```python
from build123d import *

# Parameters (mm, degrees)
THICKEN1_T2                     = 2
SURFACE_EXTRUDE1_2_DEPTH        = 65
THICKEN2_T1                     = 2
BOSS_EXTRUDE2_REACH             = 83.701
BOSS_EXTRUDE2_END_MAJOR_RADIUS  = 15
BOSS_EXTRUDE2_END_MINOR_RADIUS  = 18
BOSS_EXTRUDE2_DIRECTION_2_DEPTH = 65
SKETCH5_R                       = 1
CUT_EXTRUDE2_DEPTH              = 65
SURFACE_EXTRUDE2_3_DEPTH        = 5
THICKEN3_T1                     = 1


with BuildPart() as body_1:
    # Surface-Revolve1: a surface, the sketch's curves turned about an axis
    with BuildLine(Plane(origin=(0, 0, 0), x_dir=(1, 0, 0), z_dir=(0, 1, 0)), mode=Mode.PRIVATE) as surface_revolve1_1_path:
        Line((0, 0), (0, 15))
        ThreePointArc((0, 15), (5.857864376, 29.142135624), (20, 35))
    surface_revolve1_1 = Shell.revolve(surface_revolve1_1_path.wire(), 360, Axis((0, 0, 0), (1, 0, 0)))
    add(Solid.thicken(surface_revolve1_1, -THICKEN1_T2))

    # Surface-Extrude1: a surface, the sketch's curves swept straight by 65 mm
    with BuildLine(Plane(origin=(20, 0, 0), x_dir=(0, 0, -1), z_dir=(1, 0, 0)), mode=Mode.PRIVATE) as surface_extrude1_2_path:
        CenterArc((0, 0), 35, 0, 360)
    surface_extrude1_2 = Shell.extrude(surface_extrude1_2_path.wire(), (1 * SURFACE_EXTRUDE1_2_DEPTH, 0 * SURFACE_EXTRUDE1_2_DEPTH, 0 * SURFACE_EXTRUDE1_2_DEPTH))
    add(Solid.thicken(surface_extrude1_2, THICKEN2_T1))

    # Boss-Extrude2: up to this torus (the profile starts inside it)
    boss_extrude2_end = Plane(origin=(20, 0, 0), z_dir=(1, 0, 0)) * Torus(BOSS_EXTRUDE2_END_MAJOR_RADIUS, BOSS_EXTRUDE2_END_MINOR_RADIUS, mode=Mode.PRIVATE)
    # Sketch2 → Boss-Extrude2 (add, up to the surface)
    with BuildSketch(Plane(origin=(20, 0, 0), x_dir=(0, 0, -1), z_dir=(1, 0, 0)), mode=Mode.PRIVATE) as boss_extrude2_sk1:
        with BuildLine():
            Line((-2, 31), (-2, 33))
            Line((-2, 33), (2, 33))
            Line((2, 33), (2, 31))
            ThreePointArc((2, 31), (0, 29), (-2, 31))
        make_face()
    boss_extrude2_tool1 = extrude(boss_extrude2_sk1.sketch, amount=-BOSS_EXTRUDE2_REACH, mode=Mode.PRIVATE) & boss_extrude2_end
    add(boss_extrude2_tool1.solids().sort_by_distance((20, 31.1867, 0))[0])
    # Sketch2 → Boss-Extrude2 (add, up to the surface)
    with BuildSketch(Plane(origin=(20, 0, 0), x_dir=(0, 0, -1), z_dir=(1, 0, 0)), mode=Mode.PRIVATE) as boss_extrude2_sk2:
        with BuildLine():
            Line((-31, -2), (-33, -2))
            Line((-33, -2), (-33, 2))
            Line((-33, 2), (-31, 2))
            ThreePointArc((-31, 2), (-29, 0), (-31, -2))
        make_face()
    boss_extrude2_tool2 = extrude(boss_extrude2_sk2.sketch, amount=-BOSS_EXTRUDE2_REACH, mode=Mode.PRIVATE) & boss_extrude2_end
    add(boss_extrude2_tool2.solids().sort_by_distance((20, 0, 31.1867))[0])
    # Sketch2 → Boss-Extrude2 (add, up to the surface)
    with BuildSketch(Plane(origin=(20, 0, 0), x_dir=(0, 0, -1), z_dir=(1, 0, 0)), mode=Mode.PRIVATE) as boss_extrude2_sk3:
        with BuildLine():
            Line((2, -33), (2, -31))
            ThreePointArc((2, -31), (0, -29), (-2, -31))
            Line((-2, -31), (-2, -33))
            Line((-2, -33), (2, -33))
        make_face()
    boss_extrude2_tool3 = extrude(boss_extrude2_sk3.sketch, amount=-BOSS_EXTRUDE2_REACH, mode=Mode.PRIVATE) & boss_extrude2_end
    add(boss_extrude2_tool3.solids().sort_by_distance((20, -31.1867, 0))[0])
    # Sketch2 → Boss-Extrude2 (add, up to the surface)
    with BuildSketch(Plane(origin=(20, 0, 0), x_dir=(0, 0, -1), z_dir=(1, 0, 0)), mode=Mode.PRIVATE) as boss_extrude2_sk4:
        with BuildLine():
            Line((33, 2), (31, 2))
            ThreePointArc((31, 2), (29, 0), (31, -2))
            Line((31, -2), (33, -2))
            Line((33, -2), (33, 2))
        make_face()
    boss_extrude2_tool4 = extrude(boss_extrude2_sk4.sketch, amount=-BOSS_EXTRUDE2_REACH, mode=Mode.PRIVATE) & boss_extrude2_end
    add(boss_extrude2_tool4.solids().sort_by_distance((20, 0, -31.1867))[0])

    # Sketch2 → Boss-Extrude2 direction 2 (add)
    with BuildSketch(Plane(origin=(20, 0, 0), x_dir=(0, 0, -1), z_dir=(1, 0, 0))):
        with BuildLine():
            Line((-2, 31), (-2, 33))
            Line((-2, 33), (2, 33))
            Line((2, 33), (2, 31))
            ThreePointArc((2, 31), (0, 29), (-2, 31))
        make_face()
        with BuildLine():
            Line((-31, -2), (-33, -2))
            Line((-33, -2), (-33, 2))
            Line((-33, 2), (-31, 2))
            ThreePointArc((-31, 2), (-29, 0), (-31, -2))
        make_face()
        with BuildLine():
            Line((2, -33), (2, -31))
            ThreePointArc((2, -31), (0, -29), (-2, -31))
            Line((-2, -31), (-2, -33))
            Line((-2, -33), (2, -33))
        make_face()
        with BuildLine():
            Line((33, 2), (31, 2))
            ThreePointArc((31, 2), (29, 0), (31, -2))
            Line((31, -2), (33, -2))
            Line((33, -2), (33, 2))
        make_face()
    extrude(amount=BOSS_EXTRUDE2_DIRECTION_2_DEPTH)

    # Sketch5 → Cut-Extrude2 (cut)
    with BuildSketch(Plane(origin=(85, 0, 0), x_dir=(0, 0, -1), z_dir=(1, 0, 0))):
        with Locations((0, 31)):
            Circle(SKETCH5_R)
        with Locations((31, 0)):
            Circle(SKETCH5_R)
        with Locations((-31, 0)):
            Circle(SKETCH5_R)
        with Locations((0, -31)):
            Circle(SKETCH5_R)
    extrude(amount=-CUT_EXTRUDE2_DEPTH, mode=Mode.SUBTRACT)

    # Surface-Extrude2: a surface, the sketch's curves swept straight by 5 mm
    with BuildLine(Plane(origin=(85, 0, 0), x_dir=(0, 0, -1), z_dir=(1, 0, 0)), mode=Mode.PRIVATE) as surface_extrude2_3_path:
        CenterArc((0, 0), 35, 0, 360)
    surface_extrude2_3 = Shell.extrude(surface_extrude2_3_path.wire(), (1 * SURFACE_EXTRUDE2_3_DEPTH, 0 * SURFACE_EXTRUDE2_3_DEPTH, 0 * SURFACE_EXTRUDE2_3_DEPTH))
    add(Solid.thicken(surface_extrude2_3, THICKEN3_T1))


solid = body_1.part
```
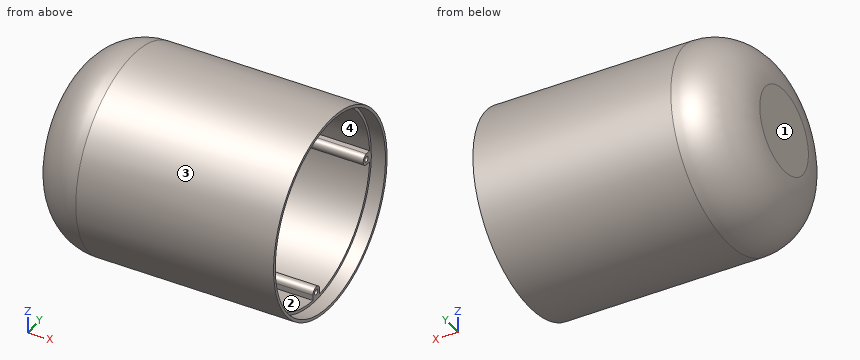
Can you work these out from the model? Positions are in its coordinate system, mm. Face numbers are marked on the shaded views. Round coordinates to 2 decimals unless told otherwise and drop trailing zeros. Loops run counter-clockwise (first coordinate to the right, second up) from the corner with the lowest first, then second, coordinate; pieces in that order, holes last. Notation, with made-up numbers: (49.25, 69.5) -> (87.25, 69.5) arc R9 ccw to (87.25, 74.5) -> close; hole circle Ø2 at (-16.5, 39). An arc over 180 degrees is marked (long way). One line per item, written item: value. Start each with the question number.
1. For pin 1 (0.6 mm diameter, centred on x = 54.5, y = -32, fed in from +Z); pin 2 (3 mm diameter, centred on x = 68.5, y = 25, fed in from +Z); pin 3 (1.5 mm diameter, centred on x = 9.5, z = -19.5, fed in from +Y), each with a flat end and sliding along its axis, tell me the tip position at first contact or that it passes through.
2. If we mould it in two halves opening along Z, with no side actions, what happens to the marked faces 1, 2, 3 and 4? For each: pulls with the +Z half, pulls with the -Z half, needs draft (parallel to the pull), parting line crosses it, or undercut.
3. If we section it at A-A, the plane x = 66: Write out the boundary of the cut face in (y, z), then the cut area to 4 significant figures.
4. If I drill on probe 1 along Y at (x, z) = (61, 0); probe 2 along Y at (x, z) = (86, 0); probe 3 along Z at (x, y) = (27.5, 23.5), over which ranges is the centre line in solid material (lowest first)?
Calculated:
1. pin 1: stops at z = 14.84
1. pin 2: stops at z = 25.94
1. pin 3: stops at y = 26.19
2. face 1: needs draft
2. face 2: undercut
2. face 3: parting line crosses it
2. face 4: undercut
3. outline: circle Ø70 at (0, 0); hole (-32.94, -2) arc R33 ccw to (-2, -32.94) -> (-2, -31) arc R2 cw to (2, -31) -> (2, -32.94) arc R33 ccw to (32.94, -2) -> (31, -2) arc R2 cw to (31, 2) -> (32.94, 2) arc R33 ccw to (2, 32.94) -> (2, 31) arc R2 cw to (-2, 31) -> (-2, 32.94) arc R33 ccw to (-32.94, 2) -> (-31, 2) arc R2 cw to (-31, -2) -> close; hole circle Ø2 at (-31, 0); hole circle Ø2 at (0, -31); hole circle Ø2 at (0, 31); hole circle Ø2 at (31, 0)
3. area: 471.5 mm²
4. probe 1: y = -35 to -32, -30 to -29, 29 to 30, 32 to 35
4. probe 2: y = -35 to -34, 34 to 35
4. probe 3: z = -25.94 to -23.17, 23.17 to 25.94
